from build123d import *

# Parameters (mm, degrees)
SKETCH2_W          = 163.5125
SKETCH2_H          = 101.6
EXTRUDE1_DEPTH     = 6.35
SKETCH3_R          = 1.524
CUT_EXTRUDE1_DEPTH = 7.35
SKETCH4_R          = 1.984375
CUT_EXTRUDE2_DEPTH = 7.35
SKETCH5_R          = 2.850007
CUT_EXTRUDE3_DEPTH = 7.35
CUT_EXTRUDE4_DEPTH = 7.35


with BuildPart() as part:
    # Sketch2 → Extrude1 (new body)
    with BuildSketch(Plane(origin=(0, 0, 0), x_dir=(1, 0, 0), z_dir=(0, 1, 0))):
        with Locations((48.149449764, -29.875011174)):
            Rectangle(SKETCH2_W, SKETCH2_H)
    extrude(amount=EXTRUDE1_DEPTH)

    # Sketch3 → Cut-Extrude1 (cut, through all)
    with BuildSketch(Plane(origin=(0, 6.35, 0), x_dir=(1, 0, 0), z_dir=(0, 1, 0))):
        with Locations(Location((-30.431800236, 17.749988826, 0), (0, 0, 270))):  # turned: the seam where the file's is
            Circle(SKETCH3_R)
        with Locations(Location((-30.431800236, -77.500011174, 0), (0, 0, 270))):  # turned: the seam where the file's is
            Circle(SKETCH3_R)
        with Locations(Location((126.730699764, -77.500011174, 0), (0, 0, 270))):  # turned: the seam where the file's is
            Circle(SKETCH3_R)
        with Locations(Location((126.730699764, 17.749988826, 0), (0, 0, 270))):  # turned: the seam where the file's is
            Circle(SKETCH3_R)
        with Locations(Location((-5.031800236, 17.749988826, 0), (0, 0, 270))):  # turned: the seam where the file's is
            Circle(SKETCH3_R)
        with Locations(Location((-5.031800236, -77.500011174, 0), (0, 0, 270))):  # turned: the seam where the file's is
            Circle(SKETCH3_R)
        with Locations(Location((101.330699764, 17.749988826, 0), (0, 0, 270))):  # turned: the seam where the file's is
            Circle(SKETCH3_R)
        with Locations(Location((101.330699764, -77.500011174, 0), (0, 0, 270))):  # turned: the seam where the file's is
            Circle(SKETCH3_R)
    extrude(amount=-CUT_EXTRUDE1_DEPTH, mode=Mode.SUBTRACT)

    # Sketch4 → Cut-Extrude2 (cut, through all)
    with BuildSketch(Plane(origin=(0, 6.35, 0), x_dir=(1, 0, 0), z_dir=(0, 1, 0))):
        with Locations(Location((7.661849764, 10.612588826, 0), (0, 0, 270))):  # turned: the seam where the file's is
            Circle(SKETCH4_R)
        with Locations(Location((88.637049764, 10.612588826, 0), (0, 0, 270))):  # turned: the seam where the file's is
            Circle(SKETCH4_R)
        with Locations(Location((7.661849764, -70.362611174, 0), (0, 0, 270))):  # turned: the seam where the file's is
            Circle(SKETCH4_R)
        with Locations(Location((88.637049764, -70.362611174, 0), (0, 0, 270))):  # turned: the seam where the file's is
            Circle(SKETCH4_R)
    extrude(amount=-CUT_EXTRUDE2_DEPTH, mode=Mode.SUBTRACT)

    # Sketch5 → Cut-Extrude3 (cut, through all)
    with BuildSketch(Plane(origin=(0, 6.35, 0), x_dir=(1, 0, 0), z_dir=(0, 1, 0))):
        with Locations(Location((48.149449764, -29.875011174, 0), (0, 0, 270))):  # turned: the seam where the file's is
            Circle(SKETCH5_R)
    extrude(amount=-CUT_EXTRUDE3_DEPTH, mode=Mode.SUBTRACT)

    # Sketch6 → Cut-Extrude4 (cut, through all)
    with BuildSketch(Plane.XZ):
        with BuildLine():
            Line((38.624449764, 5.281566926), (38.624449764, 29.875011174))
            ThreePointArc((38.624449764, 29.875011174), (48.149449764, 39.400011174), (57.674449764, 29.875011174))
            Line((57.674449764, 29.875011174), (57.674449764, 5.281566926))
            ThreePointArc((57.674449764, 5.281566926), (58.40100701, 3.947800145), (59.915626235, 3.834893734))
            ThreePointArc((59.915626235, 3.834893734), (72.157251805, 14.378041594), (76.724449764, 29.875011174))
            ThreePointArc((76.724449764, 29.875011174), (32.652480184, 53.882813215), (36.383273294, 3.834893734))
            ThreePointArc((36.383273294, 3.834893734), (37.897892519, 3.947800145), (38.624449764, 5.281566926))
        make_face()
    extrude(amount=-CUT_EXTRUDE4_DEPTH, mode=Mode.SUBTRACT)


solid = part.part
The listing builds one solid part. Answer for the finished solid, in the listing's coordinates (mm). A direction names the side the tool comes from. Give positions to 0.01 mm unless a question says otherwise; leave off trailing zeros. Write each loop counter-clockwise with the first axis right and the second up, starting at its lowest first coordinate (ties: lowest second). Pieces come first, ordered by that corner, then holes. Notation, with made-up numbers: (17.5, -29.75) -> (40.5, -29.75) arc R21 cw to (40.5, -11.75) -> close; hole circle Ø4 at (-0.75, 79). An arc over 180 degrees is marked (long way). Use a Markdown table: item, result.
(1) A flat-ended cylindrical pin translates along its axis: P1, Ø3.5, axis at x = 88.64, z = -10.61, coming from the +Y side. Find the tip coordinate at first contact, or state that the pin passes through.
Return value:
| item | result |
|---|---|
| P1 | through |
(2) Section D-D, the plane x = 55.5 is taken. Determine the outline of the cut face in (y, z).
Return value:
| item | result |
|---|---|
| outline | (0, -20.92) -> (6.35, -20.92) -> (6.35, 35.93) -> (0, 35.93) -> close; (0, 57.49) -> (6.35, 57.49) -> (6.35, 80.68) -> (0, 80.68) -> close |
(3) Section B-B, the plane y = 2.75 is taken. Give the number of separate pieces and of enclosed holes in the cut face, then the cut area to 3 significant figures.
Return value:
| item | result |
|---|---|
| separate pieces | 1 |
| enclosed holes | 14 |
| area | 14,600 mm2 |
(4) Determine the mould class of faces 3 (the flat face through (47, 0, 18)), 4 (the flat face through (129.906, 3, 31)), 5 (the cylindrical face through (-28.92, 3.22, -17.95)) for opening direction X: released by +X, released by -X, zero draft, split by the parting line, or undercut.
Return value:
| item | result |
|---|---|
| face 3 | zero draft |
| face 4 | released by +X |
| face 5 | undercut |
(5) Find the intervals of material crossed by probe 1 along X at (y, z) = (3, 10.5); probe 2 along X at (y, z) = (2.25, 29); probe 3 along Z at (x, y) = (-4.5, 4.25), in increasing order. Write a range as from..to.
Return value:
| item | result |
|---|---|
| probe 1 | -33.61..27.15, 38.62..57.67, 69.15..129.91 |
| probe 2 | -33.61..19.59, 38.62..45.44, 50.86..57.67, 76.71..129.91 |
| probe 3 | -20.92..-19.18, -16.32..76.07, 78.93..80.68 |
(6) Section C-C, the plane x = 21.5 is taken. Determine the outline of the cut face in (y, z).
Return value:
| item | result |
|---|---|
| outline | (0, -20.92) -> (6.35, -20.92) -> (6.35, 19.56) -> (0, 19.56) -> close; (0, 40.19) -> (6.35, 40.19) -> (6.35, 80.68) -> (0, 80.68) -> close |
(7) For faces 1 (the flat face through (38.624, 3, 17)), 2 (the flat face through (47, 6.35, 18)), determine the directions among +Z, -Z, +X, -X, +Y, -Y from which every point of the face is accessible in a straight line to the end or side of a thin tool.
Return value:
| item | result |
|---|---|
| face 1 | +Y, -Y |
| face 2 | +Z, -Z, +X, -X, +Y |
(8) Section A-A, the plane z = 25 is taken. Determine the outline of the cut face in (x, y), then the cut area to 3 significant figures.
Return value:
| item | result |
|---|---|
| outline | (-33.61, 0) -> (19.99, 0) -> (19.99, 6.35) -> (-33.61, 6.35) -> close; (38.62, 0) -> (57.67, 0) -> (57.67, 6.35) -> (38.62, 6.35) -> close; (76.31, 0) -> (129.91, 0) -> (129.91, 6.35) -> (76.31, 6.35) -> close |
| area | 802 mm2 |
